from build123d import *

# Parameters (mm, degrees)
SCHIZZO2_R                   = 41.625
SCHIZZO2_R_2                 = 1.3
ESTRUSIONE_ESTRUSIONE1_DEPTH = 4.15
SCHIZZO3_R                   = 2.325
TAGLIO_ESTRUSIONE1_DEPTH     = 2.15


with BuildPart() as part:
    # Schizzo1 → Rivoluzione1 (revolve)
    with BuildSketch(Plane(origin=(0, 0, 0), x_dir=(0, 0, -1), z_dir=(1, 0, 0)), mode=Mode.PRIVATE) as rivoluzione1_sk:
        Polygon((-13.885, 41.625), (13.885, 41.625), (13.885, 45.725), (14.685, 45.725), (14.685, 46.725), (11.485, 46.725), (11.485, 43.125), (6.635, 43.125), (6.635, 46.725), (4.45, 46.725), (4.45, 43.125), (-4.45, 43.125), (-4.45, 46.725), (-6.635, 46.725), (-6.635, 43.125), (-11.485, 43.125), (-11.485, 46.725), (-14.685, 46.725), (-14.685, 45.725), (-13.885, 45.725), align=None)
    revolve(rivoluzione1_sk.sketch.rotate(Axis((0, 0, 0), (0, 0, 1)), 90), axis=Axis((0, 0, 0), (0, 0, 1)))

    # Schizzo2 → Estrusione-Estrusione1 (add)
    with BuildSketch(Plane.XY.offset(3.385)):
        with Locations(Location((0, 0, 0), (0, 0, 180))):
            Circle(SCHIZZO2_R)
        with Locations(Location((0, 39, 0), (0, 0, 180))):
            Circle(SCHIZZO2_R_2, mode=Mode.SUBTRACT)
        with Locations(Location((33.774990748, 19.5, 0), (0, 0, 180))):
            Circle(SCHIZZO2_R_2, mode=Mode.SUBTRACT)
        with Locations(Location((33.774990748, -19.5, 0), (0, 0, 180))):
            Circle(SCHIZZO2_R_2, mode=Mode.SUBTRACT)
        with Locations(Location((0, -39, 0), (0, 0, 180))):
            Circle(SCHIZZO2_R_2, mode=Mode.SUBTRACT)
        with Locations(Location((-33.774990748, -19.5, 0), (0, 0, 180))):
            Circle(SCHIZZO2_R_2, mode=Mode.SUBTRACT)
        with Locations(Location((-33.774990748, 19.5, 0), (0, 0, 180))):
            Circle(SCHIZZO2_R_2, mode=Mode.SUBTRACT)
        with BuildLine():
            ThreePointArc((-36.131632771, 16.267935896), (-39.625, 0), (-36.131632771, -16.267935896))
            ThreePointArc((-36.131632771, -16.267935896), (-30.310889132, -17.5), (-32.154262138, -23.156943912))
            ThreePointArc((-32.154262138, -23.156943912), (-19.8125, -34.316256625), (-3.977370633, -39.424879808))
            ThreePointArc((-3.977370633, -39.424879808), (0, -35), (3.977370633, -39.424879808))
            ThreePointArc((3.977370633, -39.424879808), (19.8125, -34.316256625), (32.154262138, -23.156943912))
            ThreePointArc((32.154262138, -23.156943912), (30.310889132, -17.5), (36.131632771, -16.267935896))
            ThreePointArc((36.131632771, -16.267935896), (39.625, 0), (36.131632771, 16.267935896))
            ThreePointArc((36.131632771, 16.267935896), (30.310889132, 17.5), (32.154262138, 23.156943912))
            ThreePointArc((32.154262138, 23.156943912), (19.8125, 34.316256625), (3.977370633, 39.424879808))
            ThreePointArc((3.977370633, 39.424879808), (0, 35), (-3.977370633, 39.424879808))
            ThreePointArc((-3.977370633, 39.424879808), (-19.8125, 34.316256625), (-32.154262138, 23.156943912))
            ThreePointArc((-32.154262138, 23.156943912), (-30.310889132, 17.5), (-36.131632771, 16.267935896))
        make_face(mode=Mode.SUBTRACT)
    extrude(amount=ESTRUSIONE_ESTRUSIONE1_DEPTH)

    # Schizzo3 → Taglio-Estrusione1 (cut)
    with BuildSketch(Plane.XY.offset(7.535)):
        with Locations((-33.774990748, -19.5)):
            Circle(SCHIZZO3_R)
        with Locations((-33.774990748, 19.5)):
            Circle(SCHIZZO3_R)
        with Locations((0, 39)):
            Circle(SCHIZZO3_R)
        with Locations((33.774990748, 19.5)):
            Circle(SCHIZZO3_R)
        with Locations((33.774990748, -19.5)):
            Circle(SCHIZZO3_R)
        with Locations((0, -39)):
            Circle(SCHIZZO3_R)
    extrude(amount=-TAGLIO_ESTRUSIONE1_DEPTH, mode=Mode.SUBTRACT)


solid = part.part
Source: CAD feature listing. Evaluate the final solid. Frame: model axes, mm. A direction names the side the tool comes from. Coordinates: 2 decimals unless noted, no trailing zeros. Order: outer loops, then holes, each group sorted by start corner. A loop starts at its lowest first (then second) coordinate and runs counter-clockwise, first axis right, second up. Notation, with made-up numbers: M -19.5,40 L -2.5,40 A21 ccw -2.5,50 Z; hole C 74.25,42 d1. An arc over 180 degrees is marked long. Write each question's results on one line, items separated by ' | '. Start each with the question number.
Item 1: Line query: probe 1 along X at (y, z) = (-19.5, 3.9) (3 decimals); probe 2 along X at (y, z) = (21.5, 6); probe 3 along Y at (x, z) = (21, 7.75). Output: solid intervals per line, ascending.
Item 2: Draft query along X for faces 1 (the face through (34, 31, -14.685)), 2 (the face through (37.08, 28.43, -13.06)), 3 (the face through (-32.743, -18.709, 4.371)). Return one class per face: pulls with the +X half, pulls with the -X half, needs draft (parallel to the pull), parting line crosses it, or undercut.
Item 3: Cut plane B-B (x = 0). Count the separate pieces of the cut face and the enclosed holes in it, and give its area (3 significant figures).
Item 4: Cut plane A-A (z = 9). Return loops of the section in (x, y) (3 decimals), and give its area (3 significant figures).
Item 5: Set-up query: faces 4 (the face through (-33, -21, 5.385)), 5 (the face through (41, 14, 4.45)), 6 (the face through (37.08, 28.43, 13.11)). Return all of +Z, -Z, +X, -X, +Y, -Y with unobstructed straight access to the full face (end or side cutting, diameter ignored); none if empty.
Item 6: First-contact query: pin 1 Ø5.5 at (x, y) = (-33.77, -19.5) entering from +Z (3 decimals); pin 2 Ø6 at (x, z) = (21.5, 0.5) entering from -Y; pin 3 Ø6 at (x, y) = (33.77, -19.5) entering from -Z (3 decimals). Flat tips, straight axial feed; report the tip coordinate or a pass-through.
Checked values:
1) probe 1: x = -38.464 to -35.075, -32.475 to -29.775, 29.775 to 32.475, 35.075 to 38.464 | probe 2: x = -41.48 to -34.96, -32.59 to -30.31, 30.31 to 32.59, 34.96 to 41.48 | probe 3: y = -37.67 to -35.94, 35.94 to 37.67
2) face 1: needs draft | face 2: parting line crosses it | face 3: undercut
3) separate pieces: 4 | enclosed holes: 0 | area: 177 mm2
4) outline: C 0,0 d86.25; hole C 0,0 d83.25 | area: 399 mm2
5) face 4: +Z | face 5: none | face 6: +Z, -Z
6) pin 1: stops at z = 13.885 | pin 2: stops at y = -38.96 | pin 3: stops at z = -13.885
